```python
from build123d import *

# Parameters (mm, degrees)
BOSS_EXTRUDE1_DEPTH = 5
BOSS_EXTRUDE2_DEPTH = 50
CUT_EXTRUDE1_DEPTH  = 10
SKETCH6_R           = 10.25
CUT_EXTRUDE2_DEPTH  = 10
SKETCH7_R           = 10.25
CUT_EXTRUDE3_DEPTH  = 10
SKETCH8_R           = 1.6
CUT_EXTRUDE4_DEPTH  = 10
FILLET1_R           = 8
SKETCH10_W          = 80
SKETCH10_H          = 20
SKETCH10_R          = 1.6
BOSS_EXTRUDE5_DEPTH = 5
FILLET4_R           = 5
FILLET5_R           = 10


with BuildPart() as part:
    # Sketch2 → Boss-Extrude1 (new body)
    with BuildSketch(Plane(origin=(0, 0, 0), x_dir=(1, 0, 0), z_dir=(0, 1, 0))):
        Polygon((-14.142135624, 0), (0, 0), (35.355339059, 35.355339059), (85.355339059, 35.355339059), (120.710678119, 0), (134.852813742, 0), (89.497474683, 45.355339059), (31.213203436, 45.355339059), align=None)
        Polygon((85.355339059, 35.355339059), (35.355339059, 35.355339059), (0, 0), (120.710678119, 0), align=None)
    extrude(amount=BOSS_EXTRUDE1_DEPTH)

    # Sketch3 → Boss-Extrude2 (add)
    with BuildSketch(Plane(origin=(0, 5, 0), x_dir=(1, 0, 0), z_dir=(0, 1, 0))):
        Polygon((-14.142135624, 0), (31.213203436, 45.355339059), (89.497474683, 45.355339059), (134.852813742, 0), (127.781745931, 0), (87.426406871, 40.355339059), (33.284271247, 40.355339059), (-7.071067812, 0), align=None)
    extrude(amount=BOSS_EXTRUDE2_DEPTH)

    # Sketch5 → Cut-Extrude1 (cut)
    with BuildSketch(Plane(origin=(0, 0, -45.355339059), x_dir=(-1, 0, 0), z_dir=(0, 0, -1))):
        with BuildLine():
            ThreePointArc((-50.105339059, 35), (-60.355339059, 45.25), (-70.605339059, 35))
            Line((-70.605339059, 35), (-50.105339059, 35))
        make_face()
        with BuildLine():
            Line((-50.105339059, 35), (-70.605339059, 35))
            ThreePointArc((-70.605339059, 35), (-60.355339059, 24.75), (-50.105339059, 35))
        make_face()
    extrude(amount=-CUT_EXTRUDE1_DEPTH, mode=Mode.SUBTRACT)

    # Sketch6 → Cut-Extrude2 (cut)
    with BuildSketch(Plane(origin=(67.426406871, 0, -67.426406871), x_dir=(-0.7071067811865509, 0, -0.7071067811865441), z_dir=(0.7071067811865441, 0, -0.7071067811865509))):
        with Locations((-63.284271247, 35)):
            Circle(SKETCH6_R)
    extrude(amount=-CUT_EXTRUDE2_DEPTH, mode=Mode.SUBTRACT)

    # Sketch7 → Cut-Extrude3 (cut)
    with BuildSketch(Plane(origin=(-7.071067812, 0, -7.071067812), x_dir=(-0.7071067811865513, 0, 0.7071067811865438), z_dir=(-0.7071067811865438, 0, -0.7071067811865513))):
        with Locations((-22.071067812, 35)):
            Circle(SKETCH7_R)
    extrude(amount=-CUT_EXTRUDE3_DEPTH, mode=Mode.SUBTRACT)

    # Sketch8 → Cut-Extrude4 (cut)
    with BuildSketch(Plane(origin=(0, 5, 0), x_dir=(1, 0, 0), z_dir=(0, 1, 0))):
        with Locations(Location((60.355339059, 10, 0), (0, 0, 270))):
            Circle(SKETCH8_R)
        with Locations(Location((92.855339059, 10, 0), (0, 0, 270))):
            Circle(SKETCH8_R)
        with Locations(Location((27.855339059, 10, 0), (0, 0, 270))):
            Circle(SKETCH8_R)
    extrude(amount=-CUT_EXTRUDE4_DEPTH, mode=Mode.SUBTRACT)

    # Fillet1
    fillet1_edges = [part.edges().sort_by_distance(p)[0] for p in [
        (13.106601718, 5, -20.17766953),
        (60.355339059, 5, -40.355339059),
        (33.284271247, 30, -40.355339059),
        (107.604076401, 5, -20.17766953),
        (87.426406871, 30, -40.355339059),
        (60.355339059, 0, -45.355339059),
        (112.175144213, 0, -22.67766953),
        (8.535533906, 0, -22.67766953),
        (31.213203436, 27.5, -45.355339059),
        (89.497474683, 27.5, -45.355339059),
    ]]
    fillet(fillet1_edges, radius=FILLET1_R)

    # Sketch10 → Boss-Extrude5 (add)
    with BuildSketch(Plane(origin=(0, 5, 0), x_dir=(1, 0, 0), z_dir=(0, 1, 0))):
        with Locations((60.355339059, -10)):
            Rectangle(SKETCH10_W, SKETCH10_H)
        with Locations(Location((60.355339059, -15, 0), (0, 0, 270))):
            Circle(SKETCH10_R, mode=Mode.SUBTRACT)
        with Locations(Location((92.855339059, -15, 0), (0, 0, 270))):
            Circle(SKETCH10_R, mode=Mode.SUBTRACT)
        with Locations(Location((27.855339059, -15, 0), (0, 0, 270))):
            Circle(SKETCH10_R, mode=Mode.SUBTRACT)
    extrude(amount=-BOSS_EXTRUDE5_DEPTH)

    # Fillet4
    fillet4_edges = [part.edges().sort_by_distance(p)[0] for p in [
        (100.355339059, 2.5, 20),
        (100.355339059, 2.5, 0),
        (20.355339059, 2.5, 0),
        (20.355339059, 2.5, 20),
    ]]
    fillet(fillet4_edges, radius=FILLET4_R)

    # Fillet5
    # the kernel refuses this fillet: 10 mm, written as the material it takes off along each edge
    with BuildSketch(Plane(origin=(17.928932188, 55, 0), x_dir=(0, -1, 0), z_dir=(-1, 0, 0))) as fillet5_piece_1:
        with BuildLine():
            CenterArc((FILLET5_R, -FILLET5_R), FILLET5_R, 90, 90)
            Line((0, -FILLET5_R), (0, 0))
            Line((0, 0), (FILLET5_R, 0))
        make_face()
    extrude(amount=57.071067812, mode=Mode.SUBTRACT)
    with BuildSketch(Plane(origin=(159.852813742, 55, 0), x_dir=(0, 0, -1), z_dir=(-1, 0, 0))) as fillet5_piece_2:
        with BuildLine():
            CenterArc((FILLET5_R, FILLET5_R), FILLET5_R, 180, 90)
            Line((0, FILLET5_R), (0, 0))
            Line((0, 0), (FILLET5_R, 0))
        make_face()
    extrude(amount=57.071067812, mode=Mode.SUBTRACT)


solid = part.part
```
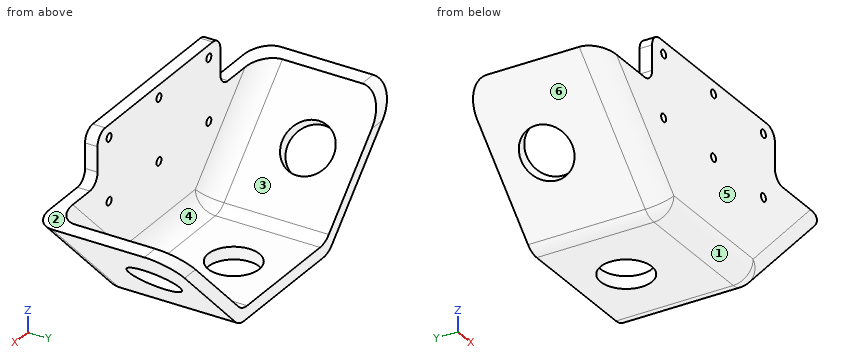
Read the model definition and answer for the solid it produces. Units are mm, in the model's axes. Face numbers are marked on the shaded views. A direction names the side the tool comes from. Give positions to 0.01 mm unless a question says otherwise; leave off trailing zeros. Write each loop counter-clockwise with the first axis right and the second up, starting at its lowest first coordinate (ties: lowest second). Pieces come first, ordered by that corner, then holes. Notation, with made-up numbers: M 35.25,-25.75 L 65.25,-25.75 A26 cw 65.25,5.25 Z; hole C 15.5,82 d3. An arc over 180 degrees is marked long. Put each result on its own line as item: value. Start each with the question number.
1. Consider line 1 along X through (y, z) = (1.3, 15); line 2 along X through (y, z) = (1.55, -10); line 3 along Y through (x, z) = (61, -29). Determine where each line is inside the solid, lowest interval first.
2. The part is cut by section D-D, the plane z = 3.5. Give the vertices of the cut face in (x, y).
3. Each of these flat-tipped pins is pushed along its axis until it touches: pin 1 Ø1.5 at (y, z) = (2, 12) entering from -X; pin 2 Ø4 at (x, y) = (39.5, 17) entering from +Z; pin 3 Ø4 at (x, z) = (21, -16.5) entering from +Y. Where does it stop, or does it pass through?
4. The part is cut by section C-C, the plane y = 23. Give the vertices of the cut face in (x, z), and give its area (3 significant figures).
5. The part is cut by section B-B, the plane y = 35. Give the vertices of the cut face in (x, z), and give its area (3 significant figures).
6. The part is cut by section A-A, the plane x = 47.5. Give the vertices of the cut face in (y, z).
7. For a pull along X with two mould halves and no side action, classify the marked faces 4, 5 and 6 as released by +X, released by -X, zero draft, split by the parting line, or undercut.
8. Which of the six approach directions +Z, -Z, +X, -X, +Y, -Y give full straight-line access (tool end or side, diameter ignored) to the marked faces 1, 2 and 3?
Final values:
1. line 1: x = 20.36 to 26.26, 29.46 to 58.76, 61.96 to 91.26, 94.46 to 100.36
1. line 2: x = 0.48 to 26.26, 29.46 to 58.76, 61.96 to 91.26, 94.46 to 120.23
1. line 3: y = 0 to 5
2. outline: M 20.13,0 L 100.59,0 L 100.59,5 L 20.13,5 Z
3. pin 1: stops at x = 20.36
3. pin 2: stops at z = -40.36
3. pin 3: stops at y = 5.21
4. outline: M -14.14,0 L 28.87,-43.01 A8 ccw 34.53,-45.36 L 86.18,-45.36 A8 ccw 91.84,-43.01 L 134.85,0 L 127.78,0 L 89.77,-38.01 A8 cw 84.11,-40.36 L 36.6,-40.36 A8 cw 30.94,-38.01 L -7.07,0 Z
4. area: 887 mm²
5. outline: M -14.14,0 L 1.29,-15.43 L 4.82,-11.89 L -7.07,0 Z; M 15.78,-29.93 L 28.87,-43.01 A8 ccw 34.53,-45.36 L 50.11,-45.36 L 50.11,-40.36 L 36.6,-40.36 A8 cw 30.94,-38.01 L 19.32,-26.39 Z; M 70.61,-45.36 L 86.18,-45.36 A8 ccw 91.84,-43.01 L 104.93,-29.93 L 101.39,-26.39 L 89.77,-38.01 A8 cw 84.11,-40.36 L 70.61,-40.36 Z; M 115.89,-11.89 L 119.42,-15.43 L 134.85,0 L 127.78,0 Z
5. area: 580 mm²
6. outline: M 0,-37.36 A8 ccw 8,-45.36 L 55,-45.36 L 55,-40.36 L 13,-40.36 A8 cw 5,-32.36 L 5,20 L 0,20 Z
7. face 4: undercut
7. face 5: zero draft
7. face 6: released by -X
8. face 1: -Z, +X, -X, -Y
8. face 2: +Z, +X, +Y, -Y
8. face 3: +Z, +Y
